Part model, mm, in its own coordinate system. Face numbers are marked on the shaded views. Give positions to 0.01 mm unless a question says otherwise; leave off trailing zeros. Write each loop counter-clockwise with the first axis right and the second up, starting at its lowest first coordinate (ties: lowest second). Pieces come first, ordered by that corner, then holes. Notation, with made-up numbers: M 89.5,-8.75 L 143.5,-8.75 A22 ccw 143.5,26.25 Z; hole C -26,74 d11. An arc over 180 degrees is marked long. Use a Markdown table: item, result. Add a question column.
from build123d import *

# Parameters (mm, degrees)
F0_W      = 90
F0_H      = 90
F1_DEPTH  = 40
F3_D      = 71
F5_D      = 5.1054
F6_D      = 6.8
F8_D      = 5
F10_D     = 8.5
F10_DEPTH = 19
F10_TIP   = 2.5536576309


# Not quite as in the source:
# - a feature names something its author has since deleted; it is built from what else it names


with BuildPart() as f1:
    # F0 (on Front) → F1 (new body)
    with BuildSketch(Plane.XZ):
        with Locations((45, 45)):
            Rectangle(F0_W, F0_H)
    extrude(amount=F1_DEPTH)

    # F3 (through all)
    with Locations(Plane.XZ.offset(40)):
        with Locations((45, 45)):
            Hole(F3_D / 2)

    # F5 (through all)
    with Locations(Plane.YZ.offset(90)):
        with Locations((-34, 45)):
            Hole(F5_D / 2)

    # F6 (through all)
    with Locations(Plane.YZ.offset(90)):
        with Locations((-20, 45)):
            Hole(F6_D / 2)

    # F8 (through all)
    with Locations(Plane.XY.offset(90)):
        with Locations((45, -34)):
            Hole(F8_D / 2)

    # F10
    with Locations(Plane.XY.offset(90)):
        with Locations((10, -20), (80, -20)):
            Hole(F10_D / 2, depth=F10_DEPTH)
            with Locations((0, 0, -(F10_DEPTH + F10_TIP / 2))):  # 118° drill point
                Cone(0, F10_D / 2, F10_TIP, mode=Mode.SUBTRACT)


solid = f1.part
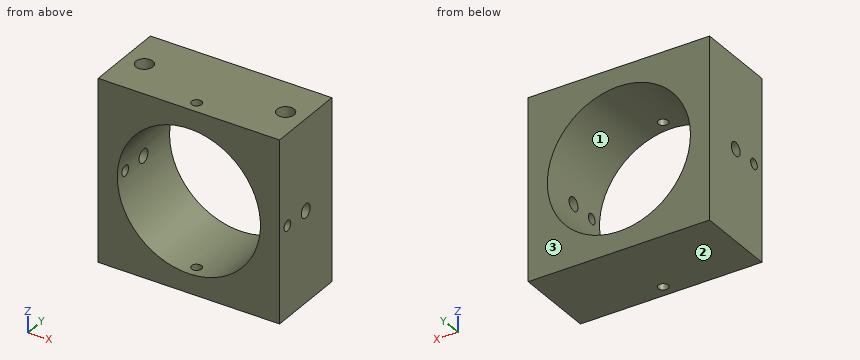
1. Mould opens along Z. For the marked faces 1, 2 and 3 say: released by +Z, released by -Z, zero draft, split by the parting line, or undercut.
2. Drill centre lines: probe 1 along Y at (x, z) = (2, 45); probe 2 along X at (y, z) = (-20, 82.5); probe 3 along Y at (x, z) = (80, 84). Where is each one in solid material? Low to high. Write a range as [from, to].
3. Cut at B-B (y = -34). Write the cut outline in (x, z).
4. Cut at D-D (z = 77). Write the cut outline in (x, y), then the cut area to 3 significant figures.
5. Flat gauge pin, fed straight in: pin 1 (4 mm diameter, centred on x = 45, y = -34, fed in from +Z) (1 decimal). Where does the tip first touch, or does it go through?
6. Cut at C-C (x = 73). Write the cut outline in (y, z), then the cut area to 3 significant figures.
7. Cut at A-A (z = 45). Write the cut outline in (x, y).
A:
| question | item | result |
|---|---|---|
| 1 | face 1 | undercut |
| 1 | face 2 | released by -Z |
| 1 | face 3 | zero draft |
| 2 | probe 1 | y = [-40, -36.55], [-31.45, -23.4], [-16.6, 0] |
| 2 | probe 2 | x = [0, 5.75], [14.25, 75.75], [84.25, 90] |
| 2 | probe 3 | y = [-40, -24.25], [-15.75, 0] |
| 3 | outline | M 0,0 L 42.5,0 L 42.5,9.59 A35.5 cw 9.59,42.45 L 0,42.45 Z; M 0,47.55 L 9.59,47.55 A35.5 cw 42.5,80.41 L 42.5,90 L 0,90 Z; M 47.5,0 L 90,0 L 90,42.45 L 80.41,42.45 A35.5 cw 47.5,9.59 Z; M 47.5,80.41 A35.5 cw 80.41,47.55 L 90,47.55 L 90,90 L 47.5,90 Z |
| 4 | outline | M 0,-40 L 29.63,-40 L 29.63,0 L 0,0 Z; M 60.37,-40 L 90,-40 L 90,0 L 60.37,0 Z; hole C 10,-20 d8.5; hole C 80,-20 d8.5 |
| 4 | area | 2,260 mm² |
| 5 | pin 1 | passes through |
| 6 | outline | M -40,0 L 0,0 L 0,23.18 L -40,23.18 Z; M -40,66.82 L 0,66.82 L 0,90 L -40,90 Z |
| 6 | area | 1,850 mm² |
| 7 | outline | M 0,-40 L 9.5,-40 L 9.5,-36.55 L 0,-36.55 Z; M 0,-31.45 L 9.5,-31.45 L 9.5,-23.4 L 0,-23.4 Z; M 0,-16.6 L 9.5,-16.6 L 9.5,0 L 0,0 Z; M 80.5,-40 L 90,-40 L 90,-36.55 L 80.5,-36.55 Z; M 80.5,-31.45 L 90,-31.45 L 90,-23.4 L 80.5,-23.4 Z; M 80.5,-16.6 L 90,-16.6 L 90,0 L 80.5,0 Z |
